The listing builds one solid part. Answer for the finished solid, in the listing's coordinates (mm). A direction names the side the tool comes from. Give positions to 0.01 mm unless a question says otherwise; leave off trailing zeros. Loops run counter-clockwise (first coordinate to the right, second up) from the corner with the lowest first, then second, coordinate; pieces in that order, holes last. Notation, with made-up numbers: (42, 67.5) - (83, 67.5) arc R26 ccw to (83, 106.5) - close; hole circle Ø6 at (22.5, 86.25). An arc over 180 degrees is marked (long way). Write each question's results on one line, items separated by ' | '.
from build123d import *

# Parameters (mm, degrees)
EXTRUDE1_DEPTH      = 28.575
CUT_EXTRUDE1_REACH  = 34.214
SKETCH2_R           = 4.0005
SKETCH2_R_2         = 1.1938
SKETCH21_R          = 4.0005
SKETCH21_R_2        = 1.1938
CUT_EXTRUDE11_DEPTH = 1.524
CUT_EXTRUDE13_REACH = 39.179
SKETCH23_W          = 41.275
SKETCH23_H          = 19.9644
CUT_EXTRUDE14_REACH = 39.179
SKETCH24_R          = 2.1844
CUT_EXTRUDE16_REACH = 41.072
SKETCH26_R          = 1.5875
SKETCH27_W          = 12.7
SKETCH27_H          = 7.9502
CUT_EXTRUDE17_DEPTH = 33.213819492
FILLET1_R           = 0.254
FILLET2_R           = 1.778
FILLET3_R           = 3.175


with BuildPart() as part:
    # Sketch1 → Extrude1 (new body, symmetric)
    with BuildSketch(Plane.XY):
        Polygon((-22.954013802, 24.902533728), (-16.2814, 0), (15.536778129, 0), (6.905111211, 32.213819492), (5.433040251, 31.819379267), (13.550662661, 1.524), (-15.11199367, 1.524), (-21.481942843, 25.296973952), align=None)
    extrude(amount=EXTRUDE1_DEPTH, both=True)

    # Sketch2 → Cut-Extrude1 (cut, up to next)
    with BuildSketch(Plane(origin=(0.432553042, 0, 10.730384283), x_dir=(-1, 0, 0), z_dir=(0, 1, 0)), mode=Mode.PRIVATE) as cut_extrude1_sk1:
        with Locations(Location((0.432553042, -2.399184283, 0), (0, 0, 270))):  # turned: the seam where the file's is
            Circle(SKETCH2_R)
    cut_extrude1_tool1 = extrude(cut_extrude1_sk1.sketch, amount=CUT_EXTRUDE1_REACH, mode=Mode.PRIVATE) & part.part
    add(cut_extrude1_tool1.solids().sort_by_distance((0, 0, 8.3312))[0], mode=Mode.SUBTRACT)
    # Sketch2 → Cut-Extrude1 (cut, up to next)
    with BuildSketch(Plane(origin=(0.432553042, 0, 10.730384283), x_dir=(-1, 0, 0), z_dir=(0, 1, 0)), mode=Mode.PRIVATE) as cut_extrude1_sk2:
        with Locations(Location((0.432553042, 5.932015717, 0), (0, 0, 270))):  # turned: the seam where the file's is
            Circle(SKETCH2_R_2)
    cut_extrude1_tool2 = extrude(cut_extrude1_sk2.sketch, amount=CUT_EXTRUDE1_REACH, mode=Mode.PRIVATE) & part.part
    add(cut_extrude1_tool2.solids().sort_by_distance((0, 0, 16.6624))[0], mode=Mode.SUBTRACT)
    # Sketch2 → Cut-Extrude1 (cut, up to next)
    with BuildSketch(Plane(origin=(0.432553042, 0, 10.730384283), x_dir=(-1, 0, 0), z_dir=(0, 1, 0)), mode=Mode.PRIVATE) as cut_extrude1_sk3:
        with Locations(Location((8.763753042, -2.399184283, 0), (0, 0, 270))):  # turned: the seam where the file's is
            Circle(SKETCH2_R_2)
    cut_extrude1_tool3 = extrude(cut_extrude1_sk3.sketch, amount=CUT_EXTRUDE1_REACH, mode=Mode.PRIVATE) & part.part
    add(cut_extrude1_tool3.solids().sort_by_distance((-8.3312, 0, 8.3312))[0], mode=Mode.SUBTRACT)
    # Sketch2 → Cut-Extrude1 (cut, up to next)
    with BuildSketch(Plane(origin=(0.432553042, 0, 10.730384283), x_dir=(-1, 0, 0), z_dir=(0, 1, 0)), mode=Mode.PRIVATE) as cut_extrude1_sk4:
        with Locations(Location((0.432553042, -10.730384283, 0), (0, 0, 270))):  # turned: the seam where the file's is
            Circle(SKETCH2_R_2)
    cut_extrude1_tool4 = extrude(cut_extrude1_sk4.sketch, amount=CUT_EXTRUDE1_REACH, mode=Mode.PRIVATE) & part.part
    add(cut_extrude1_tool4.solids().sort_by_distance((0, 0, 0))[0], mode=Mode.SUBTRACT)
    # Sketch2 → Cut-Extrude1 (cut, up to next)
    with BuildSketch(Plane(origin=(0.432553042, 0, 10.730384283), x_dir=(-1, 0, 0), z_dir=(0, 1, 0)), mode=Mode.PRIVATE) as cut_extrude1_sk5:
        with Locations(Location((-7.898646958, -2.399184283, 0), (0, 0, 270))):  # turned: the seam where the file's is
            Circle(SKETCH2_R_2)
    cut_extrude1_tool5 = extrude(cut_extrude1_sk5.sketch, amount=CUT_EXTRUDE1_REACH, mode=Mode.PRIVATE) & part.part
    add(cut_extrude1_tool5.solids().sort_by_distance((8.3312, 0, 8.3312))[0], mode=Mode.SUBTRACT)

    # Sketch21 → Cut-Extrude11 (cut)
    with BuildSketch(Plane(origin=(1.025651892, 0, -16.036287214), x_dir=(-1, 0, 0), z_dir=(0, 1, 0))):
        with Locations(Location((1.025651892, 7.705087214, 0), (0, 0, 270))):  # turned: the seam where the file's is
            Circle(SKETCH21_R)
        with Locations(Location((1.025651892, 16.036287214, 0), (0, 0, 270))):  # turned: the seam where the file's is
            Circle(SKETCH21_R_2)
        with Locations(Location((9.356851892, 7.705087214, 0), (0, 0, 270))):  # turned: the seam where the file's is
            Circle(SKETCH21_R_2)
        with Locations(Location((1.025651892, -0.626112786, 0), (0, 0, 270))):  # turned: the seam where the file's is
            Circle(SKETCH21_R_2)
        with Locations(Location((-7.305548108, 7.705087214, 0), (0, 0, 270))):  # turned: the seam where the file's is
            Circle(SKETCH21_R_2)
    extrude(amount=CUT_EXTRUDE11_DEPTH, mode=Mode.SUBTRACT)

    # Sketch23 → Cut-Extrude13 (cut, up to next)
    with BuildSketch(Plane(origin=(14.496011341, 3.884194532, 0), x_dir=(0, 0, -1), z_dir=(0.965925826, 0.258819045, 0)), mode=Mode.PRIVATE) as cut_extrude13_sk1:
        with Locations((0.0127, 19.346785921)):
            Rectangle(SKETCH23_W, SKETCH23_H)
    cut_extrude13_tool1 = extrude(cut_extrude13_sk1.sketch, amount=-CUT_EXTRUDE13_REACH, mode=Mode.PRIVATE) & part.part
    add(cut_extrude13_tool1.solids().sort_by_distance((9.488695, 22.571755, -0.0127))[0], mode=Mode.SUBTRACT)

    # Sketch24 → Cut-Extrude14 (cut, up to next)
    with BuildSketch(Plane(origin=(14.496011341, 3.884194532, 0), x_dir=(0, 0, -1), z_dir=(0.965925826, 0.258819045, 0)), mode=Mode.PRIVATE) as cut_extrude14_sk1:
        with Locations(Location((-24.4094, 24.274385921, 0), (0, 0, 90))):  # turned: the seam where the file's is
            Circle(SKETCH24_R)
    cut_extrude14_tool1 = extrude(cut_extrude14_sk1.sketch, amount=-CUT_EXTRUDE14_REACH, mode=Mode.PRIVATE) & part.part
    add(cut_extrude14_tool1.solids().sort_by_distance((8.213338, 27.331451, 24.4094))[0], mode=Mode.SUBTRACT)
    # Sketch24 → Cut-Extrude14 (cut, up to next)
    with BuildSketch(Plane(origin=(14.496011341, 3.884194532, 0), x_dir=(0, 0, -1), z_dir=(0.965925826, 0.258819045, 0)), mode=Mode.PRIVATE) as cut_extrude14_sk2:
        with Locations(Location((-24.4094, 14.444585921, 0), (0, 0, 90))):  # turned: the seam where the file's is
            Circle(SKETCH24_R)
    cut_extrude14_tool2 = extrude(cut_extrude14_sk2.sketch, amount=-CUT_EXTRUDE14_REACH, mode=Mode.PRIVATE) & part.part
    add(cut_extrude14_tool2.solids().sort_by_distance((10.757477, 17.836593, 24.4094))[0], mode=Mode.SUBTRACT)
    # Sketch24 → Cut-Extrude14 (cut, up to next)
    with BuildSketch(Plane(origin=(14.496011341, 3.884194532, 0), x_dir=(0, 0, -1), z_dir=(0.965925826, 0.258819045, 0)), mode=Mode.PRIVATE) as cut_extrude14_sk3:
        with Locations(Location((24.7904, 24.274385921, 0), (0, 0, 90))):  # turned: the seam where the file's is
            Circle(SKETCH24_R)
    cut_extrude14_tool3 = extrude(cut_extrude14_sk3.sketch, amount=-CUT_EXTRUDE14_REACH, mode=Mode.PRIVATE) & part.part
    add(cut_extrude14_tool3.solids().sort_by_distance((8.213338, 27.331451, -24.7904))[0], mode=Mode.SUBTRACT)
    # Sketch24 → Cut-Extrude14 (cut, up to next)
    with BuildSketch(Plane(origin=(14.496011341, 3.884194532, 0), x_dir=(0, 0, -1), z_dir=(0.965925826, 0.258819045, 0)), mode=Mode.PRIVATE) as cut_extrude14_sk4:
        with Locations(Location((24.7904, 14.444585921, 0), (0, 0, 90))):  # turned: the seam where the file's is
            Circle(SKETCH24_R)
    cut_extrude14_tool4 = extrude(cut_extrude14_sk4.sketch, amount=-CUT_EXTRUDE14_REACH, mode=Mode.PRIVATE) & part.part
    add(cut_extrude14_tool4.solids().sort_by_distance((10.757477, 17.836593, -24.7904))[0], mode=Mode.SUBTRACT)

    # Sketch26 → Cut-Extrude16 (cut, up to next)
    with BuildSketch(Plane(origin=(-15.190753005, -4.07035, 0), x_dir=(0, 0, 1), z_dir=(-0.965925826, -0.258819045, 0)), mode=Mode.PRIVATE) as cut_extrude16_sk1:
        with Locations(Location((-11.5062, 20.063536401, 0), (0, 0, 270))):  # turned: the seam where the file's is
            Circle(SKETCH26_R)
    cut_extrude16_tool1 = extrude(cut_extrude16_sk1.sketch, amount=-CUT_EXTRUDE16_REACH, mode=Mode.PRIVATE) & part.part
    add(cut_extrude16_tool1.solids().sort_by_distance((-20.383578, 15.309538, -11.5062))[0], mode=Mode.SUBTRACT)
    # Sketch26 → Cut-Extrude16 (cut, up to next)
    with BuildSketch(Plane(origin=(-15.190753005, -4.07035, 0), x_dir=(0, 0, 1), z_dir=(-0.965925826, -0.258819045, 0)), mode=Mode.PRIVATE) as cut_extrude16_sk2:
        with Locations(Location((11.5062, 20.063536401, 0), (0, 0, 270))):  # turned: the seam where the file's is
            Circle(SKETCH26_R)
    cut_extrude16_tool2 = extrude(cut_extrude16_sk2.sketch, amount=-CUT_EXTRUDE16_REACH, mode=Mode.PRIVATE) & part.part
    add(cut_extrude16_tool2.solids().sort_by_distance((-20.383578, 15.309538, 11.5062))[0], mode=Mode.SUBTRACT)

    # Sketch27 → Cut-Extrude17 (cut, through all)
    with BuildSketch(Plane.XZ):
        with Locations((-21.46199367, 24.5999)):
            Rectangle(SKETCH27_W, SKETCH27_H)
        with Locations((-21.46199367, -24.5999)):
            Rectangle(SKETCH27_W, SKETCH27_H)
    extrude(amount=-CUT_EXTRUDE17_DEPTH, mode=Mode.SUBTRACT)

    # Fillet1
    fillet1_edges = [part.edges().sort_by_distance(p)[0] for p in [
        (-15.11199367, 1.524, 0),
        (13.550662661, 1.524, 0),
    ]]
    fillet(fillet1_edges, radius=FILLET1_R)

    # Fillet2
    fillet2_edges = [part.edges().sort_by_distance(p)[0] for p in [
        (15.536778129, 0, 0),
        (-16.2814, 0, 0),
    ]]
    fillet(fillet2_edges, radius=FILLET2_R)

    # Fillet3
    fillet3_edges = [part.edges().sort_by_distance(p)[0] for p in [
        (-22.217978322, 25.09975384, 20.6248),
        (-22.217978322, 25.09975384, -20.6248),
        (6.169075731, 32.01659938, 28.575),
        (6.169075731, 32.01659938, -28.575),
    ]]
    fillet(fillet3_edges, radius=FILLET3_R)


solid = part.part
Item 1: A cutting plane is placed at A-A, the plane z = 0. Determine the outline of the cut face in (x, y), plus the area to 3 significant figures.
Values found:
outline: (-22.95, 24.9) - (-16.63, 1.32) arc R1.78 ccw to (-14.92, 0) - (-1.19, 0) - (-1.19, 1.52) - (-14.92, 1.52) arc R0.25 cw to (-15.16, 1.71) - (-21.48, 25.3) - close; (1.19, 0) - (13.22, 0) arc R1.78 ccw to (14.94, 2.24) - (12.07, 12.93) - (10.6, 12.54) - (13.46, 1.84) arc R0.25 cw to (13.22, 1.52) - (1.19, 1.52) - close | area: 98.2 mm²
Item 2: A cutting plane is placed at C-C, the plane y = 21. Determine the outline of the cut face in (x, z) (3 decimals), plus the area to 3 significant figures.
Values found:
outline: (-21.908, -20.625) - (-20.331, -20.625) - (-20.331, 20.625) - (-21.908, 20.625) - close; (8.332, -28.575) - (9.91, -28.575) - (9.91, -20.65) - (8.332, -20.65) - close; (8.332, 20.625) - (9.91, 20.625) - (9.91, 28.575) - (8.332, 28.575) - close | area: 90.1 mm²
Item 3: Flat-ended cylindrical pins translate along their axes: P1, Ø4, axis at x = -8.33, z = -8.33, coming from the +Y side; P2, Ø2, axis at y = 11, z = -2, coming from the +X side; P3, Ø3, axis at y = 8.5, z = -1.5, coming from the +X side. Find the tip coordinate at first contact, or state that the pin passes through.
Values found:
P1: stops at y = 1.52 | P2: stops at x = 12.86 | P3: stops at x = 13.66
Item 4: A cutting plane is placed at D-D, the plane z = -14. Determine the outline of the cut face in (x, y).
Values found:
outline: (-22.95, 24.9) - (-16.63, 1.32) arc R1.78 ccw to (-14.92, 0) - (13.22, 0) arc R1.78 ccw to (14.94, 2.24) - (12.07, 12.93) - (10.6, 12.54) - (13.46, 1.84) arc R0.25 cw to (13.22, 1.52) - (-14.92, 1.52) arc R0.25 cw to (-15.16, 1.71) - (-21.48, 25.3) - close
Item 5: Find the intervals of material crossed by line 1 along Y through (x, z) = (-1, 12.5); line 2 along X through (y, z) = (5, 20.5); line 3 along X through (y, z) = (7.5, 11), in increasing order. Write a range as [from, to].
Values found:
line 1: y = [0, 1.52] | line 2: x = [-17.62, -16.04], [12.62, 14.2] | line 3: x = [-18.29, -16.71], [11.95, 13.53]
Item 6: For faces 5 (the face through (-4, 1.524, 0)), 6 (the face through (10.597, 15.534, -24.694)), determine the directions among +Z, -Z, +X, -X, +Y, -Y from which every point of the face is accessible in a straight line to the end or side of a thin tool.
Values found:
face 5: +Z, -Z | face 6: none
Item 7: For a pull along Z with two mould halves and no side action, classify faces 1 (the face through (6.18, 32.02, 23.05)), 2 (the face through (1.532, 0.751, -12.027)), 3 (the face through (-21.994, 24.222, -19.67)), 4 (the face through (-19.98, 16.72, 10.54)) as released by +Z, released by -Z, zero draft, split by the parting line, or undercut.
Values found:
face 1: zero draft | face 2: undercut | face 3: released by -Z | face 4: undercut
Item 8: A cutting plane is placed at B-B, the plane x = 0. Determine the outline of the cut face in (y, z) (3 decimals), plus the area to 3 significant figures.
Values found:
outline: (0, -28.575) - (1.524, -28.575) - (1.524, -17.856) - (0, -17.856) - close; (0, -15.469) - (1.524, -15.469) - (1.524, -12.332) - (0, -12.332) - close; (0, -4.331) - (1.524, -4.331) - (1.524, -1.194) - (0, -1.194) - close; (0, 1.194) - (1.524, 1.194) - (1.524, 4.331) - (0, 4.331) - close; (0, 12.332) - (1.524, 12.332) - (1.524, 15.469) - (0, 15.469) - close; (0, 17.856) - (1.524, 17.856) - (1.524, 28.575) - (0, 28.575) - close | area: 51.8 mm²
